Geometry: final body of the model. Coordinates: model frame, mm. Give positions to 0.01 mm unless a question says otherwise; leave off trailing zeros. Loops run counter-clockwise (first coordinate to the right, second up) from the corner with the lowest first, then second, coordinate; pieces in that order, holes last.
from build123d import *

# Parameters (mm, degrees)
F0_R     = 2.683726
F1_DEPTH = 4.572


with BuildPart() as f1:
    # F0 (on Front) → F1 (new body)
    with BuildSketch(Plane.XZ):
        with BuildLine():
            Line((25.310985, -22.970802), (28.093947, -18.754418))
            Line((28.093947, -18.754418), (17.928825, -12.04508))
            Line((17.928825, -12.04508), (17.243224, -13.083814))
            add(Edge.make_bspline(
                [(14.305283, -11.253849), (14.527919, -13.088348), (16.233271, -13.663207), (17.243224, -13.083814)],
                knots=[0, 0, 0, 0, 3.461252, 3.461252, 3.461252, 3.461252], degree=3))
            Line((14.305283, -11.253849), (10.843506, -16.498686))
            Line((10.843506, -16.498686), (21.512225, -23.540416))
            add(Edge.make_bspline(
                [(21.512225, -23.540416), (22.463378, -23.924239), (23.950653, -23.793526), (25.310985, -22.970802)],
                knots=[0, 0, 0, 0, 3.841229, 3.841229, 3.841229, 3.841229], degree=3))
        make_face()
        with Locations((22.88826, -19.738317)):
            Circle(F0_R, mode=Mode.SUBTRACT)
    extrude(amount=F1_DEPTH)


solid = f1.part
Item 1: Section query A-A on z = -17.5. Return loops of the section in (x, y), plus the area to 3 significant figures.
Values follow:
outline: (12.36, -4.57) - (21.41, -4.57) - (21.41, 0) - (12.36, 0) - close; (24.37, -4.57) - (26.19, -4.57) - (26.19, 0) - (24.37, 0) - close
area: 49.7 mm2
Item 2: Section query C-C on x = 13.5. Return loops of the section in (y, z), plus the area to 3 significant figures.
Values follow:
outline: (-4.57, -18.25) - (0, -18.25) - (0, -12.47) - (-4.57, -12.47) - close
area: 26.4 mm2
Item 3: Pin query (flat end, axial travel): pin 1 (1 mm diameter, centred on y = -1.5, z = -20.5, fed in from -X). Return the tip coordinate at first contact, or that it passes through.
Values follow:
pin 1: stops at x = 16.15
Item 4: Ray query, probe 1 along Z at (x, y) = (21.5, -0.7); probe 2 along X at (y, z) = (-1.7, -18.25); probe 3 along X at (y, z) = (-0.55, -12.5). Return the intervals inside material, ascending.
Values follow:
probe 1: z = -23.53 to -22.04, -17.44 to -14.4
probe 2: x = 13.5 to 20.66, 25.12 to 27.33
probe 3: x = 13.48 to 14.79, 17.63 to 18.62
Item 5: Section query B-B on z = -19. Return loops of the section in (x, y).
Values follow:
outline: (14.63, -4.57) - (20.31, -4.57) - (20.31, 0) - (14.63, 0) - close; (25.47, -4.57) - (27.93, -4.57) - (27.93, 0) - (25.47, 0) - close
Item 6: Section query D-D on z = -14. Return loops of the section in (x, y).
Values follow:
outline: (12.49, -4.57) - (20.89, -4.57) - (20.89, 0) - (12.49, 0) - close
Item 7: Draft query along X for faces 1 (the face through (17.59, -2.25, -12.56)), 2 (the face through (16.1, -2.25, -19.97)), 3 (the face through (19, 0, -18)). Return one class per face: +X half, -X half, draft (parallel to the pull), parting line (faces both ways), or undercut.
Values follow:
face 1: undercut
face 2: -X half
face 3: draft
